from build123d import *

# Parameters (mm, degrees)
SKETCH1_R                  = 25.4
EXTRUDE1_DEPTH             = 50.8
F_1_2_0_5_DIAMETER_HOLE1_D = 12.7254
CHAMFER1_SIZE              = 0.762
F_1_1_DIAMETER_HOLE1_D     = 25.4
F_1_1_DIAMETER_HOLE1_DEPTH = 42.418
CHAMFER2_SIZE              = 0.254
CHAMFER3_SIZE              = 0.635


with BuildPart() as part:
    # Sketch1 → Extrude1 (new body)
    with BuildSketch(Plane(origin=(0, 0, 0), x_dir=(1, 0, 0), z_dir=(0, 1, 0))):
        with Locations(Location((0, 0, 0), (0, 0, 270))):  # turned: the seam where the file's is
            Circle(SKETCH1_R)
    extrude(amount=EXTRUDE1_DEPTH)

    # 1/2 (0.5) Diameter Hole1 (through all)
    with Locations(Plane(origin=(0, 50.8, 0), x_dir=(-1, 0, 0), z_dir=(0, 1, 0))):
        with Locations((0, 0)):
            Hole(F_1_2_0_5_DIAMETER_HOLE1_D / 2)

    # Chamfer1
    chamfer1_edges = [part.edges().sort_by_distance(p)[0] for p in [
        (0, 0, -25.4),
        (0, 50.8, -25.4),
        (-6.3627, 0, 0),
    ]]
    chamfer(chamfer1_edges, length=CHAMFER1_SIZE)

    # 1 (1) Diameter Hole1
    with Locations(Plane(origin=(0, 50.8, 0), x_dir=(-1, 0, 0), z_dir=(0, 1, 0))):
        with Locations((0, 0)):
            Hole(F_1_1_DIAMETER_HOLE1_D / 2, depth=F_1_1_DIAMETER_HOLE1_DEPTH)

    # Chamfer2
    chamfer2_edges = [part.edges().sort_by_distance(p)[0] for p in [
        (-12.7, 8.382, 0),
    ]]
    chamfer(chamfer2_edges, length=CHAMFER2_SIZE)

    # Chamfer3
    chamfer3_edges = [part.edges().sort_by_distance(p)[0] for p in [
        (-12.7, 50.8, 0),
    ]]
    chamfer(chamfer3_edges, length=CHAMFER3_SIZE)


solid = part.part
Model file for the job. Use its own axes, mm. A direction names the side the tool comes from. Coordinates: 2 decimals unless noted, no trailing zeros. Order: outer loops, then holes, each group sorted by start corner. A loop starts at its lowest first (then second) coordinate and runs counter-clockwise, first axis right, second up. Notation, with made-up numbers: M -12,29.25 L 26,29.25 A21 ccw 26,55.25 Z; hole C 61,-15.75 d10. An arc over 180 degrees is marked long. Return JSON: item names as keys, results as strings.
1. Drill centre lines: probe 1 along Z at (x, y) = (-11.5, 36.5); probe 2 along Y at (x, z) = (0, -7.5); probe 3 along X at (y, z) = (28, 7). Where is each one in solid material? Low to high.
Ans:
{"probe 1": "-22.65 to -5.39, 5.39 to 22.65", "probe 2": "0 to 8.38", "probe 3": "-24.42 to -10.6, 10.6 to 24.42"}
2. Saw through at A-A (z = 0). Give the cut face in (x, y) (3 decimals).
Ans:
{"outline": "M -25.4,0.762 L -24.638,0 L -7.125,0 L -6.363,0.762 L -6.363,8.382 L -12.446,8.382 L -12.7,8.636 L -12.7,50.165 L -13.335,50.8 L -24.638,50.8 L -25.4,50.038 Z; M 6.363,0.762 L 7.125,0 L 24.638,0 L 25.4,0.762 L 25.4,50.038 L 24.638,50.8 L 13.335,50.8 L 12.7,50.165 L 12.7,8.636 L 12.446,8.382 L 6.363,8.382 Z"}
3. Saw through at B-B (x = 0). Give the cut face in (y, z) (3 decimals), and give its area (3 significant figures).
Ans:
{"outline": "M 0,-24.638 L 0.762,-25.4 L 50.038,-25.4 L 50.8,-24.638 L 50.8,-13.335 L 50.165,-12.7 L 8.636,-12.7 L 8.382,-12.446 L 8.382,-6.363 L 0.762,-6.363 L 0,-7.125 Z; M 0,7.125 L 0.762,6.363 L 8.382,6.363 L 8.382,12.446 L 8.636,12.7 L 50.165,12.7 L 50.8,13.335 L 50.8,24.638 L 50.038,25.4 L 0.762,25.4 L 0,24.638 Z", "area": "1,390 mm^2"}
4. Flat gauge pins, fed straight in: pin 1 (3 mm diameter, centred on y = 40.5, z = -5.5, fed in from +X); pin 2 (1.5 mm diameter, centred on y = 24, z = 11, fed in from +X); pin 3 (6 mm diameter, centred on y = 42, z = 5.5, fed in from -X). Where does each tip first touch, or does it go through?
Ans:
{"pin 1": "x = 25.08", "pin 2": "x = 23.24", "pin 3": "x = -25.28"}
5. Saw through at C-C (y = 13). Give the cut face in (x, z).
Ans:
{"outline": "C 0,0 d50.8; hole C 0,0 d25.4"}
6. Pull direction X, two halves, no side cores. Call faces 1 (the face through (-0.83, 4.52, 6.31)), 2 (the face through (-15.456, 25.055, -20.157)), 3 (the face through (-11, 50.8, 11)): +X half, -X half, draft (parallel to the pull), parting line (faces both ways), or undercut.
Ans:
{"face 1": "undercut", "face 2": "parting line", "face 3": "draft"}
7. Tool access for faces 4 (the face through (-6, 8.382, 3)), 5 (the face through (6, 0, 5)): list every direction of +Z, -Z, +X, -X, +Y, -Y with a clear straight run to the whole face (end or side of a thin tool).
Ans:
{"face 4": "+Y", "face 5": "+Z, -Z, +X, -X, -Y"}
